Part model, mm, in its own coordinate system. A direction names the side the tool comes from. Round coordinates to 2 decimals unless told otherwise and drop trailing zeros. Loops run counter-clockwise (first coordinate to the right, second up) from the corner with the lowest first, then second, coordinate; pieces in that order, holes last.
Autodesk Inventor part; units mm, degrees
ref_plane "Work Plane1" through (0, 0, 15.875) normal (0, 0, 1) x (1, 0, 0)
ref_plane "YZ Plane" through (0, 0, 0) normal (1, 0, 0) x (0, 1, 0)
ref_plane "XZ Plane" through (0, 0, 0) normal (0, 1, 0) x (-1, 0, 0)
sketch "Sketch1" plane through (0, 0, 0) normal (0, 0, 1) x (1, 0, 0)
  line L0 (0, 0) -> (539.75, 0)
  line L1 (539.75, 0) -> (539.75, 168.275)
  line L2 (539.75, 168.275) -> (0, 168.275)
  line L3 (0, 168.275) -> (0, 0)
  dimension "d0" = 539.75
  dimension "d1" = 168.275
extrude "Extrusion1" add sketch "Sketch1" along normal blind 25.4
sketch "Sketch2" plane through (0, 0, 25.4) normal (0, 0, 1) x (1, 0, 0)
  line L0 (539.75, 0) -> (539.75, 168.275)
  line L1 (0, 168.275) -> (0, 0)
  line L2 (0, 168.275) -> (539.75, 168.275)
  line L3 (539.75, 168.275) -> (539.75, 120.65)
  line L4 (539.75, 120.65) -> (0, 120.65)
  line L5 (0, 120.65) -> (0, 168.275)
  line L6 (0, 107.95) -> (539.75, 107.95)
  line L7 (539.75, 107.95) -> (539.75, 60.325)
  line L8 (539.75, 60.325) -> (0, 60.325)
  line L9 (0, 60.325) -> (0, 107.95)
  line L10 (0, 47.625) -> (539.75, 47.625)
  line L11 (539.75, 47.625) -> (539.75, 0)
  line L12 (539.75, 0) -> (0, 0)
  line L13 (0, 0) -> (0, 47.625)
  line L14 (0, 120.65) -> (539.75, 120.65)
  line L15 (539.75, 120.65) -> (539.75, 107.95)
  line L16 (539.75, 107.95) -> (0, 107.95)
  line L17 (0, 107.95) -> (0, 120.65)
  line L18 (539.75, 60.325) -> (0, 60.325)
  line L19 (0, 60.325) -> (0, 47.625)
  line L20 (0, 47.625) -> (539.75, 47.625)
  line L21 (539.75, 47.625) -> (539.75, 60.325)
  dimension "d4" = 47.625
  dimension "d5" = 47.625
  dimension "d6" = 47.625
  dimension "d7" = 12.7
  dimension "d8" = 12.7
extrude "Extrusion3" cut sketch "Sketch2" against normal blind 19.05 contours L10 L1 L8 L0 | L6 L1 L4 L0
sketch "Sketch3" plane through (0, 0, 25.4) normal (0, 0, 1) x (1, 0, 0)
  line L0 (0, 120.65) -> (539.75, 120.65)
  line L1 (539.75, 120.65) -> (539.75, 168.275)
  line L2 (539.75, 168.275) -> (0, 168.275)
  line L3 (0, 168.275) -> (0, 120.65)
  line L4 (0, 155.575) -> (539.75, 155.575)
  line L5 (539.75, 155.575) -> (539.75, 146.05)
  line L6 (539.75, 146.05) -> (0, 146.05)
  line L7 (0, 146.05) -> (0, 155.575)
  line L8 (0, 107.95) -> (558.8, 107.95)
  line L9 (558.8, 107.95) -> (558.8, 60.325)
  line L10 (558.8, 60.325) -> (0, 60.325)
  line L11 (0, 60.325) -> (0, 107.95)
  line L12 (1.6074, 47.625) -> (558.8, 47.625)
  line L13 (558.8, 47.625) -> (558.8, 0)
  line L14 (558.8, 0) -> (1.6074, 0)
  line L15 (1.6074, 0) -> (1.6074, 47.625)
  line L16 (0, 95.25) -> (558.8, 95.25)
  line L17 (558.8, 95.25) -> (558.8, 85.725)
  line L18 (558.8, 85.725) -> (0, 85.725)
  line L19 (0, 85.725) -> (0, 95.25)
  line L20 (11.1324, 34.925) -> (404.8324, 34.925)
  line L21 (404.8324, 34.925) -> (404.8324, 25.4)
  line L22 (404.8324, 25.4) -> (11.1324, 25.4)
  line L23 (11.1324, 25.4) -> (11.1324, 34.925)
  line L24 (558.8, 47.625) -> (414.3574, 47.625)
  line L25 (414.3574, 47.625) -> (414.3574, 0)
  line L26 (414.3574, 0) -> (558.8, 0)
  line L27 (558.8, 0) -> (558.8, 47.625)
  point P0 (0, 0)
  dimension "d13" = 9.525
  dimension "d14" = 12.7
  dimension "d15" = 25.4
  dimension "d16" = 12.7
  dimension "d17" = 12.7
  dimension "d18" = 47.625
  dimension "d19" = 47.625
  dimension "d20" = 9.525
  dimension "d21" = 12.7
  dimension "d22" = 393.7
  dimension "d23" = 412.75
  dimension "d24" = 9.525
  dimension "d25" = 9.525
  dimension "d26" = 9.525
  dimension "d27" = 12.7
  dimension "d28" = 539.75
ref_plane "Work Plane1" through (0, 0, 15.875) normal (0, 0, 1) x (1, 0, 0)
sketch "Sketch5" plane through (0, 0, 15.875) normal (0, 0, 1) x (1, 0, 0)
  line L0 (539.75, 47.625) -> (539.75, 0)
  line L1 (414.3574, 47.625) -> (539.75, 47.625)
  line L2 (414.3574, 0) -> (414.3574, 47.625)
  line L3 (539.75, 0) -> (414.3574, 0)
  point P0 (0, 0)
extrude "Extrusion5" cut sketch "Sketch5" against normal blind 9.525
extrude "Extrusion7" cut sketch "Sketch3" against normal blind 9.525 contours L3 L4 L1 L6 | L16 L9 L18 L11 | L12 L13 L14 L25 | L20 L21 L22 L23
equation "\"d7\" = d8"
equation "\"d19\" = d18"
equation "\"d24\" = d25"
properties part number "ply75_bottom_board" material "Wood (Cherry)"
1) Drop flat-ended pins along their axis: pin 1 Ø5.5 at (y, z) = (28.5, 11.5) entering from +X; pin 2 Ø4 at (x, y) = (216.5, 116) entering from +Z. Give the stop position or say it passes through.
Values:
pin 1: stops at x = 414.36
pin 2: stops at z = 6.35
2) Slice it at C-C, the plane x = 395.5. Give the cut face in (y, z) (3 decimals), then the cut area to 3 significant figures.
Values:
outline: (0, 0) - (168.275, 0) - (168.275, 25.4) - (155.575, 25.4) - (155.575, 15.875) - (146.05, 15.875) - (146.05, 25.4) - (120.65, 25.4) - (120.65, 6.35) - (107.95, 6.35) - (107.95, 25.4) - (95.25, 25.4) - (95.25, 15.875) - (85.725, 15.875) - (85.725, 25.4) - (60.325, 25.4) - (60.325, 6.35) - (47.625, 6.35) - (47.625, 25.4) - (34.925, 25.4) - (34.925, 15.875) - (25.4, 15.875) - (25.4, 25.4) - (0, 25.4) - close
area: 3,520 mm2
3) Tool access for faces 4 (the face through (211, 25.4, 21)), 5 (the face through (266, 73, 25.4)), 6 (the face through (204, 47.625, 16)): list every direction of +Z, -Z, +X, -X, +Y, -Y with a clear straight run to the whole face (end or side of a thin tool).
Values:
face 4: +Z
face 5: +Z, +X, -X, +Y, -Y
face 6: +Z, +X, -X
4) Slice it at A-A, the plane z = 10.5. Give the cut face in (x, y) (3 decimals), then the cut area to 3 significant figures.
Values:
outline: (0, 0) - (414.357, 0) - (414.357, 47.625) - (0, 47.625) - close; (0, 60.325) - (539.75, 60.325) - (539.75, 107.95) - (0, 107.95) - close; (0, 120.65) - (539.75, 120.65) - (539.75, 168.275) - (0, 168.275) - close
area: 71,100 mm2
5) Slice it at B-B, the plane x = 484. Give the cut face in (y, z) (3 decimals), then the cut area to 3 significant figures.
Values:
outline: (0, 0) - (168.275, 0) - (168.275, 25.4) - (155.575, 25.4) - (155.575, 15.875) - (146.05, 15.875) - (146.05, 25.4) - (120.65, 25.4) - (120.65, 6.35) - (107.95, 6.35) - (107.95, 25.4) - (95.25, 25.4) - (95.25, 15.875) - (85.725, 15.875) - (85.725, 25.4) - (60.325, 25.4) - (60.325, 6.35) - (0, 6.35) - close
area: 2,700 mm2
6) Mould opens along Y. For faces 1 (the face through (266, 155.575, 21)), 2 (the face through (266, 85, 0)), 3 (the face through (274, 168.275, 13)) say: released by +Y, released by -Y, zero draft, split by the parting line, or undercut.
Values:
face 1: undercut
face 2: zero draft
face 3: released by +Y
7) Wall check: line 1 along Y through (x, z) = (508.5, 17.5) (3 decimals); line 2 along Y through (x, z) = (248, 24.25) (3 decimals); line 3 along Y through (x, z) = (215.5, 13.25) (3 decimals). Give the ranges that are in metal, low to high.
Values:
line 1: y = 60.325 to 85.725, 95.25 to 107.95, 120.65 to 146.05, 155.575 to 168.275
line 2: y = 0 to 25.4, 34.925 to 47.625, 60.325 to 85.725, 95.25 to 107.95, 120.65 to 146.05, 155.575 to 168.275
line 3: y = 0 to 47.625, 60.325 to 107.95, 120.65 to 168.275
